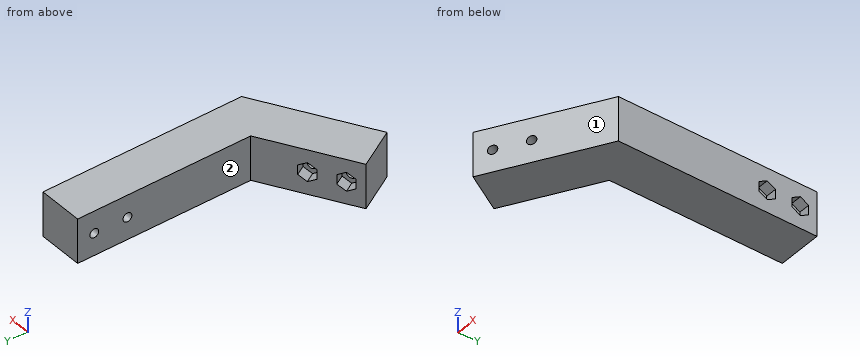
```python
from build123d import *

# Parameters (mm, degrees)
SKETCH4_W          = 20
SKETCH4_H          = 20
CUT_EXTRUDE1_REACH = 118.478
SKETCH5_R          = 2
SKETCH5_3_R        = 2
CUT_EXTRUDE2_DEPTH = 5
SKETCH6_R          = 2
CUT_EXTRUDE3_DEPTH = 139.877964102
SKETCH6_5_R        = 2
CUT_EXTRUDE4_DEPTH = 5


with BuildPart() as part:
    # Sweep1: sweep along a path in Sketch1
    with BuildLine(Plane.XY) as sweep1_path:
        Line((0, 0), (43.301270189, 25))
        Line((43.301270189, 25), (43.301270189, 109))
    # Sketch4 → Sweep1 (sweep)
    with BuildSketch(Plane(origin=(0, 0, 0), x_dir=(0, 0, 1), z_dir=(-0.866025403784438, -0.5000000000000012, 0))):
        Rectangle(SKETCH4_W, SKETCH4_H)
    sweep(path=sweep1_path.line, transition=Transition.RIGHT)

    # Sketch5 → Cut-Extrude1 (cut, up to next)
    with BuildSketch(Plane(origin=(-5, 8.660254038, 0), x_dir=(0.866025403784438, 0.5000000000000012, 0), z_dir=(-0.5000000000000012, 0.866025403784438, 0)), mode=Mode.PRIVATE) as cut_extrude1_sk1:
        with Locations(Location((7.5, 0, 0), (0, 0, 180))):
            Circle(SKETCH5_R)
    cut_extrude1_tool1 = extrude(cut_extrude1_sk1.sketch, amount=-CUT_EXTRUDE1_REACH, mode=Mode.PRIVATE) & part.part
    # Sketch5 → Cut-Extrude1 (cut, up to next)
    with BuildSketch(Plane(origin=(-5, 8.660254038, 0), x_dir=(0.866025403784438, 0.5000000000000012, 0), z_dir=(-0.5000000000000012, 0.866025403784438, 0)), mode=Mode.PRIVATE) as cut_extrude1_sk2:
        with Locations(Location((22.5, 0, 0), (0, 0, 180))):
            Circle(SKETCH5_R)
    cut_extrude1_tool2 = extrude(cut_extrude1_sk2.sketch, amount=-CUT_EXTRUDE1_REACH, mode=Mode.PRIVATE) & part.part
    add(cut_extrude1_tool1.solids().sort_by_distance((1.495191, 12.410254, 0))[0], mode=Mode.SUBTRACT)
    add(cut_extrude1_tool2.solids().sort_by_distance((14.485572, 19.910254, 0))[0], mode=Mode.SUBTRACT)

    # Sketch5<3> → Cut-Extrude2 (cut)
    # profile 1 of 2: a face of its own
    with BuildSketch(Plane(origin=(-5, 8.660254038, 0), x_dir=(0.866025403784438, 0.5000000000000012, 0), z_dir=(-0.5000000000000012, 0.866025403784438, 0))):
        Polygon((11.2, -2.136195996), (11.2, 2.136195996), (7.5, 4.272391992), (3.8, 2.136195996), (3.8, -2.136195996), (7.5, -4.272391992), align=None)
        with Locations(Location((7.5, 0, 0), (0, 0, 180))):
            Circle(SKETCH5_3_R, mode=Mode.SUBTRACT)
    # profile 2 of 2: a face of its own
    with BuildSketch(Plane(origin=(-5, 8.660254038, 0), x_dir=(0.866025403784438, 0.5000000000000012, 0), z_dir=(-0.5000000000000012, 0.866025403784438, 0))):
        Polygon((26.2, -2.136195996), (26.2, 2.136195996), (22.5, 4.272391992), (18.8, 2.136195996), (18.8, -2.136195996), (22.5, -4.272391992), align=None)
        with Locations(Location((22.5, 0, 0), (0, 0, 180))):
            Circle(SKETCH5_3_R, mode=Mode.SUBTRACT)
    extrude(amount=-CUT_EXTRUDE2_DEPTH, mode=Mode.SUBTRACT)

    # Sketch6 → Cut-Extrude3 (cut, through all)
    with BuildSketch(Plane(origin=(53.301270189, 0, -53.301270189), x_dir=(0, 0, 1), z_dir=(-1, 0, 0))):
        with Locations(Location((53.301270189, 101.5, 0), (0, 0, 90))):
            Circle(SKETCH6_R)
        with Locations(Location((53.301270189, 86.5, 0), (0, 0, 90))):
            Circle(SKETCH6_R)
    extrude(amount=CUT_EXTRUDE3_DEPTH, mode=Mode.SUBTRACT)

    # Sketch6<5> → Cut-Extrude4 (cut)
    # profile 1 of 2: a face of its own
    with BuildSketch(Plane(origin=(53.301270189, 0, -53.301270189), x_dir=(0, 0, 1), z_dir=(-1, 0, 0))):
        Polygon((55.437466185, 97.8), (57.573662181, 101.5), (55.437466185, 105.2), (51.165074193, 105.2), (49.028878197, 101.5), (51.165074193, 97.8), align=None)
        with Locations(Location((53.301270189, 101.5, 0), (0, 0, 90))):
            Circle(SKETCH6_5_R, mode=Mode.SUBTRACT)
    # profile 2 of 2: a face of its own
    with BuildSketch(Plane(origin=(53.301270189, 0, -53.301270189), x_dir=(0, 0, 1), z_dir=(-1, 0, 0))):
        Polygon((55.437466185, 82.8), (57.573662181, 86.5), (55.437466185, 90.2), (51.165074193, 90.2), (49.028878197, 86.5), (51.165074193, 82.8), align=None)
        with Locations(Location((53.301270189, 86.5, 0), (0, 0, 90))):
            Circle(SKETCH6_5_R, mode=Mode.SUBTRACT)
    extrude(amount=CUT_EXTRUDE4_DEPTH, mode=Mode.SUBTRACT)


solid = part.part
```
The model under review builds one solid part; all positions refer to its coordinate system, in mm. Face numbers are marked on the shaded views. A direction names the side the tool comes from. Give positions to 0.01 mm unless a question says otherwise; leave off trailing zeros. Write each loop counter-clockwise with the first axis right and the second up, starting at its lowest first coordinate (ties: lowest second). Pieces come first, ordered by that corner, then holes. Notation, with made-up numbers: M -7,-0.5 L 10,-0.5 A18 ccw 10,26.5 Z; hole C 51,28 d10. An arc over 180 degrees is marked long. Answer in a Markdown table with one row per item.
Item 1: Add section A-A on z = 8.5. Give the boundary of the cut face in (x, y).
Check sheet entries:
| item | result |
|---|---|
| outline | M -5,8.66 L 5,-8.66 L 53.3,19.23 L 53.3,109 L 33.3,109 L 33.3,30.77 Z |
Item 2: For line 1 along Z through (x, y) = (43, 101.5); line 2 along X through (y, z) = (14, -0.5); line 3 along Y through (x, z) = (43, 0.25), list the stretches that pass through material, from the lowest coordinate up.
Check sheet entries:
| item | result |
|---|---|
| line 1 | -10 to -2, 2 to 10 |
| line 2 | 4.85 to 13.63, 14.25 to 15.66, 20.13 to 44.25 |
| line 3 | 13.28 to 84.52, 88.48 to 99.52, 103.48 to 109 |
Item 3: Add section B-B on y = 64. Give the boundary of the cut face in (x, z).
Check sheet entries:
| item | result |
|---|---|
| outline | M 33.3,-10 L 53.3,-10 L 53.3,10 L 33.3,10 Z |
Item 4: Add section D-D on x = 28. Give the boundary of the cut face in (y, z).
Check sheet entries:
| item | result |
|---|---|
| outline | M 4.62,-10 L 27.71,-10 L 27.71,10 L 4.62,10 Z |
Item 5: For P1, Ø1.5, axis at x = 32.5, z = 3.5, coming from the -Y side; P2, Ø3, axis at x = 17.5, z = -7, coming from the -Y side; P3, Ø5, axis at y = 5.5, z = -4, coming from the +X side; P4, Ø2.5, axis at y = 86.5, z = 0, coming from the +X side, all flat-tipped, find the tip position at first contact; note any pin that passes through.
Check sheet entries:
| item | result |
|---|---|
| P1 | y = 6.78 |
| P2 | y = -2.31 |
| P3 | x = 33.86 |
| P4 | through |
Item 6: Add section C-C on z = 0. State how many separate pieces and enclosed holes the cut face has, plus the area to 3 significant figures.
Check sheet entries:
| item | result |
|---|---|
| separate pieces | 5 |
| enclosed holes | 0 |
| area | 2,290 mm2 |
Item 7: Tool access review of the marked faces 1 and 2: name each direction out of +Z, -Z, +X, -X, +Y, -Y from which nothing blocks a thin tool from reaching the whole face with its end or side.
Check sheet entries:
| item | result |
|---|---|
| face 1 | +Z, -Z, +X, -Y |
| face 2 | +Z, -Z, -X, +Y |
